Part print with two shaded views. Sizes in mm from the minimum x, y, z corner. A direction names the side the tool comes from. Coordinates: 2 decimals unless noted, no trailing zeros. Loops run counter-clockwise (first coordinate to the right, second up) from the corner with the lowest first, then second, coordinate; pieces in that order, holes last. Notation, with made-up numbers: (71.5, 87.25) - (114.5, 87.25) arc R23 cw to (114.5, 101.25) - close; hole circle Ø5 at (7, 63.25). An arc over 180 degrees is marked (long way). Answer as CSV lines item,"result".
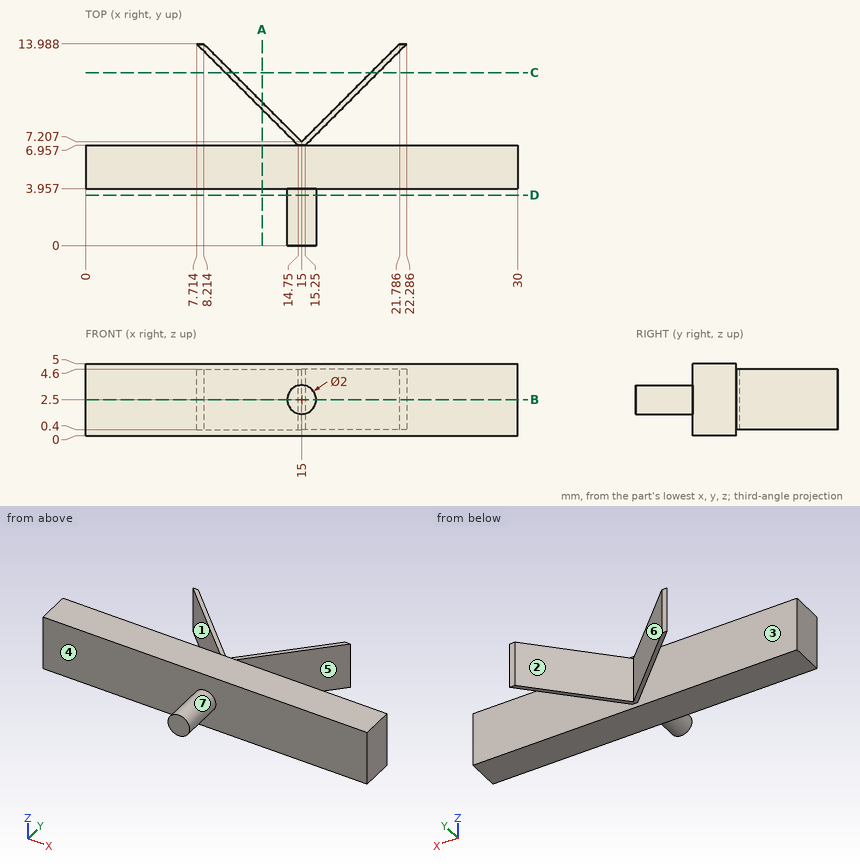
Q1. Saw through at B-B (z = 2.5). Give the cut face in (x, y), then the cut area to 3 significant figures.
Results:
outline,"(0, 3.96) - (14, 3.96) - (14, 0) - (16, 0) - (16, 3.96) - (30, 3.96) - (30, 6.96) - (15.25, 6.96) - (22.29, 13.99) - (21.79, 13.99) - (15, 7.21) - (8.21, 13.99) - (7.71, 13.99) - (14.75, 6.96) - (0, 6.96) - close"
area,"105 mm^2"
Q2. Saw through at C-C (y = 12). Give the cut face in (x, z).
Results:
outline,"(9.7, 0.4) - (10.2, 0.4) - (10.2, 4.6) - (9.7, 4.6) - close; (19.8, 0.4) - (20.3, 0.4) - (20.3, 4.6) - (19.8, 4.6) - close"
Q3. Flat gauge pins, fed straight in: pin 1 (4 mm diameter, centred on x = 17.5, y = 10, fed in from -Z); pin 2 (1.5 mm diameter, centred on x = 19.5, z = 2, fed in from -Y); pin 3 (3 mm diameter, centred on x = 10.5, z = 3.5, fed in from +Y). Where does each tip first touch, or does it go through?
Results:
pin 1,"stops at z = 0.4"
pin 2,"stops at y = 3.96"
pin 3,"stops at y = 13.2"
Q4. Wall check: L1, parallel to Y at x = 15.5, z = 4 (1 decimal); L2, parallel to Y at x = 16, z = 0.7 (1 decimal); L3, parallel to X at y = 10.5, z = 3.7 (1 decimal). Give the ranges that are in metal, low to high.
Results:
L1,"y = 4 to 7, 7.2 to 7.7"
L2,"y = 4 to 7, 7.7 to 8.2"
L3,"x = 11.2 to 11.7, 18.3 to 18.8"
Q5. Which spindle directions (+Z, -Z, +X, -X, +Y, -Y) get a long thin tool onto all of the face, cutting with end or side? Do the marked faces 5, 6 and 7. Say none if no direction does.
Results:
face 5,"+Z, -Z, +X"
face 6,"+Z, -Z, +Y"
face 7,"-Y"
Q6. Saw through at D-D (y = 3.5). Give the cut face in (x, z).
Results:
outline,"circle Ø2 at (15, 2.5)"
Q7. Two-plate mould, pull along Y, no slides. Class the marked faces 1, 2, 3 and 4: released by +Y, released by -Y, zero draft, split by the parting line, or undercut.
Results:
face 1,"undercut"
face 2,"released by +Y"
face 3,"undercut"
face 4,"released by -Y"
Q8. Saw through at A-A (x = 12.25). Give the cut face in (y, z) (1 decimal).
Results:
outline,"(4, 0) - (7, 0) - (7, 5) - (4, 5) - close; (9.5, 0.4) - (10, 0.4) - (10, 4.6) - (9.5, 4.6) - close"
